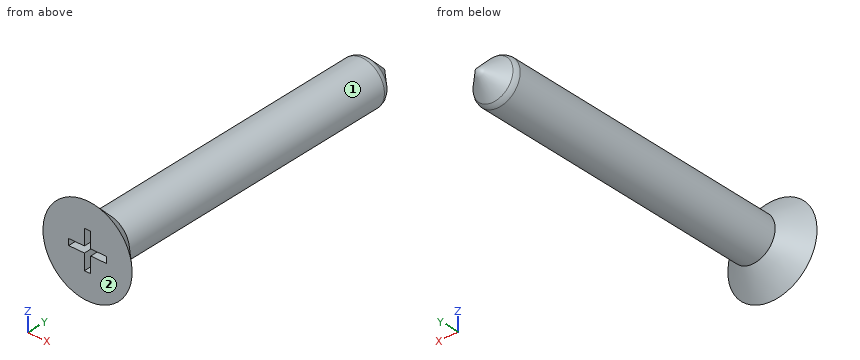
Autodesk Inventor part; units mm, degrees
ref_plane "YZ Plane" through (0, 0, 0) normal (1, 0, 0) x (0, 1, 0)
ref_plane "XZ Plane" through (0, 0, 0) normal (0, 1, 0) x (-1, 0, 0)
ref_plane "XY Plane" through (0, 0, 0) normal (0, 0, 1) x (1, 0, 0)
sketch "Sketch1" plane through (0, 0, 0) normal (1, 0, 0) x (0, 1, 0)
  line L0 (0, 0) -> (10, 0)
  line L1 (0, 0) -> (-10, 0)
  line L2 (10, 0) -> (8.5858, 1.4142)
  line L3 (8.5858, 1.4142) -> (-10, 1.4142)
  line L4 (-10, 1.4142) -> (-10, 0)
  line L5 (-10, 1.4142) -> (-11.453, 1.4142) construction
  line L6 (-10, 1.4142) -> (-11.4142, 2.8284)
  line L7 (-10, 0) -> (-12.8284, 0)
  line L8 (-11.4142, 2.8284) -> (-11.4142, 0)
  dimension "d0" = 10
  dimension "d1" = 10
  dimension "d2" = 2
  dimension "d3" = 45
  dimension "d4" = 2
  dimension "d8" = 45
revolve "Revolution1" add sketch "Sketch1" angle 360 about axis through (0, 0, 0) along (0, 1, 0)
fillet "Fillet1" radius 0.5 1 edges at (0, 8.5858, -1.4142)
sketch "Sketch3" plane through (0, -11.4142, 0) normal (0, -1, 0) x (1, 0, 0)
  line L0 (0.2, 1.2) -> (-0.2, 1.2)
  line L1 (-0.2, 1.2) -> (-0.2, -1.2)
  line L2 (-0.2, -1.2) -> (0.2, -1.2)
  line L3 (0.2, -1.2) -> (0.2, 1.2)
  line L4 (1.2, 0.2) -> (-1.2, 0.2)
  line L5 (-1.2, 0.2) -> (-1.2, -0.2)
  line L6 (-1.2, -0.2) -> (1.2, -0.2)
  line L7 (1.2, -0.2) -> (1.2, 0.2)
  point P0 (0, 0)
  dimension "d28" = 0.2
  dimension "d29" = 0.2
  dimension "d30" = 1.2
  dimension "d31" = 1.2
  dimension "d32" = 1.2
  dimension "d33" = 1.2
  dimension "d34" = 0.2
  dimension "d35" = 0.2
extrude "Extrusion1" cut sketch "Sketch3" against normal blind 1.25
thread "Thread2"
properties part number "screw"
Input: part model. Units: mm. Frame: model coordinates. Face numbers are marked on the shaded views. A direction names the side the tool comes from. Coordinates: 2 decimals unless noted, no trailing zeros. Write each loop counter-clockwise with the first axis right and the second up, starting at its lowest first coordinate (ties: lowest second). Pieces come first, ordered by that corner, then holes.
1) Pin query (flat end, axial travel): pin 1 Ø1.1 at (y, z) = (-10.5, -1) entering from +X; pin 2 Ø2 at (y, z) = (0, -2) entering from +X; pin 3 Ø0.8 at (x, y) = (1, -11) entering from -Z. Return the tip coordinate at first contact, or that it passes through.
2) Section A-A on y = 8. Output: boundary loops of the cut face in (x, z).
3) Set-up query: the marked faces 1 and 2. Return all of +Z, -Z, +X, -X, +Y, -Y with unobstructed straight access to the full face (end or side cutting, diameter ignored); none if empty.
4) Material intervals for line 1 along X through (y, z) = (-8.5, 0.75); line 2 along Y through (x, z) = (0.1, 1.8); line 3 along Y through (x, z) = (-0.65, 0.5), sorted ascending.
Check result:
1. pin 1: stops at x = 2.29
1. pin 2: stops at x = 1
1. pin 3: stops at z = -2.65
2. outline: circle Ø2.83 at (0, 0)
3. face 1: +Y
3. face 2: +Z, -Z, +X, -X, -Y
4. line 1: x = -1.2 to 1.2
4. line 2: y = -11.41 to -10.39
4. line 3: y = -11.41 to 9.18
